Work out the finished part from the listing and answer in its coordinate system (mm). A direction names the side the tool comes from. Round coordinates to 2 decimals unless told otherwise and drop trailing zeros. Order: outer loops, then holes, each group sorted by start corner. A loop starts at its lowest first (then second) coordinate and runs counter-clockwise, first axis right, second up. Notation, with made-up numbers: (-19.75, -23.75) - (24.25, -23.75) arc R28 cw to (24.25, -0.75) - close; hole circle Ø1 at (86, 79.25). An arc over 180 degrees is marked (long way). One line per question, with ' | ' between items. Start each with the question number.
from build123d import *

# Parameters (mm, degrees)
F0_W     = 18
F0_H     = 25.530076
F1_DEPTH = 3.333333


with BuildPart() as f1:
    # F0 (on Top) → F1 (new body)
    with BuildSketch(Plane.XY):
        Polygon((-46.258066, 26.794441), (-46.258066, 52.324517), (-46.258066, 56.824517), (-50.758066, 56.824517), (-50.758066, 26.794441), align=None)
        with Locations((-37.258066, 39.559479)):
            Rectangle(F0_W, F0_H)
        Polygon((-28.258066, 56.824517), (-28.258066, 52.324517), (-28.258066, 26.794441), (-23.758066, 26.794441), (-23.758066, 56.824517), align=None)
    extrude(amount=F1_DEPTH)


solid = f1.part
1) For faces 1 (the flat face through (-46.258, 55, 2)), 2 (the flat face through (-48, 56.825, 2)), determine the directions among +Z, -Z, +X, -X, +Y, -Y from which every point of the face is accessible in a straight line to the end or side of a thin tool.
2) Determine the mould class of faces 3 (the flat face through (-50.758, 42, 2)), 4 (the flat face through (-26, 56.825, 2)), 5 (the flat face through (-37, 52.325, 2)), 6 (the flat face through (-28.258, 55, 2)) for opening direction X: released by +X, released by -X, zero draft, split by the parting line, or undercut.
3) Section C-C on x = -33.5 is taken. Give the vertices of the cut face in (y, z), and give its area (3 significant figures).
4) Section B-B on z = 0.55 is taken. Give the vertices of the cut face in (x, y).
5) A flat-ended cylindrical pin translates along its axis: pin 1 (10 mm diameter, centred on x = -41.5, y = 33, fed in from -Z). Find the tip coordinate at first contact, or state that the pin passes through.
6) Section A-A on y = 55.5 is taken. Give the vertices of the cut face in (x, z).
7) Straight lines are drawn through the part: line 1 (Y direction, x = -43.25, z = 1.05); line 2 (X direction, y = 53, z = 1.8). For each, find the intervals that lie inside material, in ascending order.
Recorded:
1) face 1: +Z, -Z, +Y | face 2: +Z, -Z, +X, -X, +Y
2) face 3: released by -X | face 4: zero draft | face 5: undercut | face 6: undercut
3) outline: (26.79, 0) - (52.32, 0) - (52.32, 3.33) - (26.79, 3.33) - close | area: 85.1 mm²
4) outline: (-50.76, 26.79) - (-23.76, 26.79) - (-23.76, 56.82) - (-28.26, 56.82) - (-28.26, 52.32) - (-46.26, 52.32) - (-46.26, 56.82) - (-50.76, 56.82) - close
5) pin 1: stops at z = 0
6) outline: (-50.76, 0) - (-46.26, 0) - (-46.26, 3.33) - (-50.76, 3.33) - close; (-28.26, 0) - (-23.76, 0) - (-23.76, 3.33) - (-28.26, 3.33) - close
7) line 1: y = 26.79 to 52.32 | line 2: x = -50.76 to -46.26, -28.26 to -23.76
